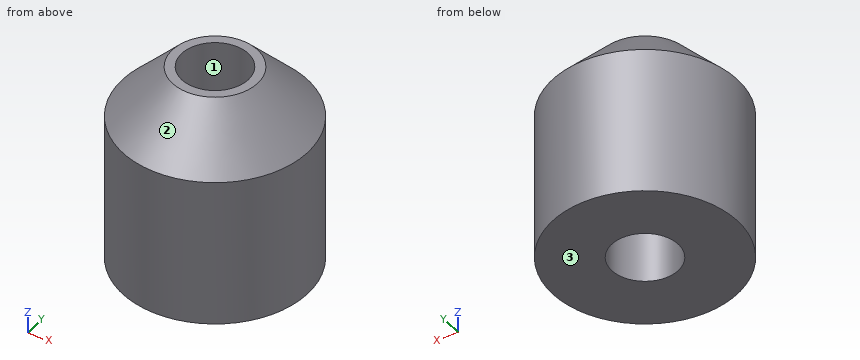
from build123d import *

# Parameters (mm, degrees)
CYLINDER100_R     = 1.8
CYLINDER100_DEPTH = 2.8
TUBE_R            = 5
TUBE_R_2          = 1.8
TUBE_DEPTH        = 8


with BuildPart() as puller_washer_cone_hole:
    # Cylinder100 → Cylinder100 (new body)
    with BuildSketch(Plane.XY):
        Circle(CYLINDER100_R)
    extrude(amount=CYLINDER100_DEPTH)


with BuildPart() as puller_washer_cone_cut:
    # Cone → Cone (revolve)
    with BuildSketch(Plane.XZ):
        Polygon((0, 0), (5, 0), (2.3, 2.8), (0, 2.8), align=None)
    revolve(axis=Axis((0, 0, 0), (0, 0, 1)))

    # Cut: cut puller washer cone hole
    add(puller_washer_cone_hole.part, mode=Mode.SUBTRACT)


with BuildPart() as puller_washer_cone_cut_1:
    # Cut placement: moved
    add(puller_washer_cone_cut.part.moved(Location((0, 0, 8))))


with BuildPart() as puller_mount_washer:
    # Tube → Tube (new body)
    with BuildSketch(Plane.XY):
        Circle(TUBE_R)
        Circle(TUBE_R_2, mode=Mode.SUBTRACT)
    extrude(amount=TUBE_DEPTH)

    # Fusion: union puller washer cone cut
    add(puller_washer_cone_cut_1.part)


solid = puller_mount_washer.part
Work out the finished part from the listing and answer in its coordinate system (mm). Face numbers are marked on the shaded views. Round coordinates to 2 decimals unless told otherwise and drop trailing zeros. Order: outer loops, then holes, each group sorted by start corner. A loop starts at its lowest first (then second) coordinate and runs counter-clockwise, first axis right, second up. Notation, with made-up numbers: M 4.25,54.5 L 28.25,54.5 A14 cw 28.25,78.5 Z; hole C 22.5,14 d8. An arc over 180 degrees is marked long. Put each result on its own line as item: value. Start each with the question number.
Q1. Section C-C, the plane z = 9 is taken. Write down the section's boundary in (x, y).
Q2. Section A-A, the plane x = 0 is taken. Write down the section's boundary in (y, z), and give its area (3 significant figures).
Q3. For a pull along X with two mould halves and no side action, classify the marked faces 1, 2 and 3 as pulls with the +X half, pulls with the -X half, needs draft (parallel to the pull), parting line crosses it, or undercut.
Q4. Straight lines are drawn through the part: L1, parallel to Y at x = 0, z = 2.5; L2, parallel to X at y = 0.25, z = 3.75; L3, parallel to X at y = -1.25, z = 9.5. For each, find the intervals that lie inside material, in ascending order. Write a range as [from, to].
Q5. Section B-B, the plane z = 3 is taken. Write down the section's boundary in (x, y), and give its area (3 significant figures).
Q6. Flat-ended cylindrical pins translate along their axes: pin 1 (1.5 mm diameter, centred on y = -2.5, z = 6, fed in from +X); pin 2 (1 mm diameter, centred on y = -1, z = 2, fed in from +X); pin 3 (4 mm diameter, centred on y = 3.5, z = 8, fed in from +X). Find the tip coordinate at first contact, or state that the pin passes through.
Findings below:
1. outline: C 0,0 d8.07; hole C 0,0 d3.6
2. outline: M -5,0 L -1.8,0 L -1.8,10.8 L -2.3,10.8 L -5,8 Z; M 1.8,0 L 5,0 L 5,8 L 2.3,10.8 L 1.8,10.8 Z
2. area: 61.6 mm^2
3. face 1: undercut
3. face 2: parting line crosses it
3. face 3: needs draft
4. L1: y = [-5, -1.8], [1.8, 5]
4. L2: x = [-4.99, -1.78], [1.78, 4.99]
4. L3: x = [-3.33, -1.3], [1.3, 3.33]
5. outline: C 0,0 d10; hole C 0,0 d3.6
5. area: 68.4 mm^2
6. pin 1: stops at x = 4.68
6. pin 2: stops at x = 4.97
6. pin 3: stops at x = 4.77
